Answer from the drawing. Dimensions are ordinates in mm from the lowest x, y and z of the part. A direction names the side the tool comes from. Coordinates: 2 decimals unless noted, no trailing zeros. Loops run counter-clockwise (first coordinate to the right, second up) from the corner with the lowest first, then second, coordinate; pieces in that order, holes last.
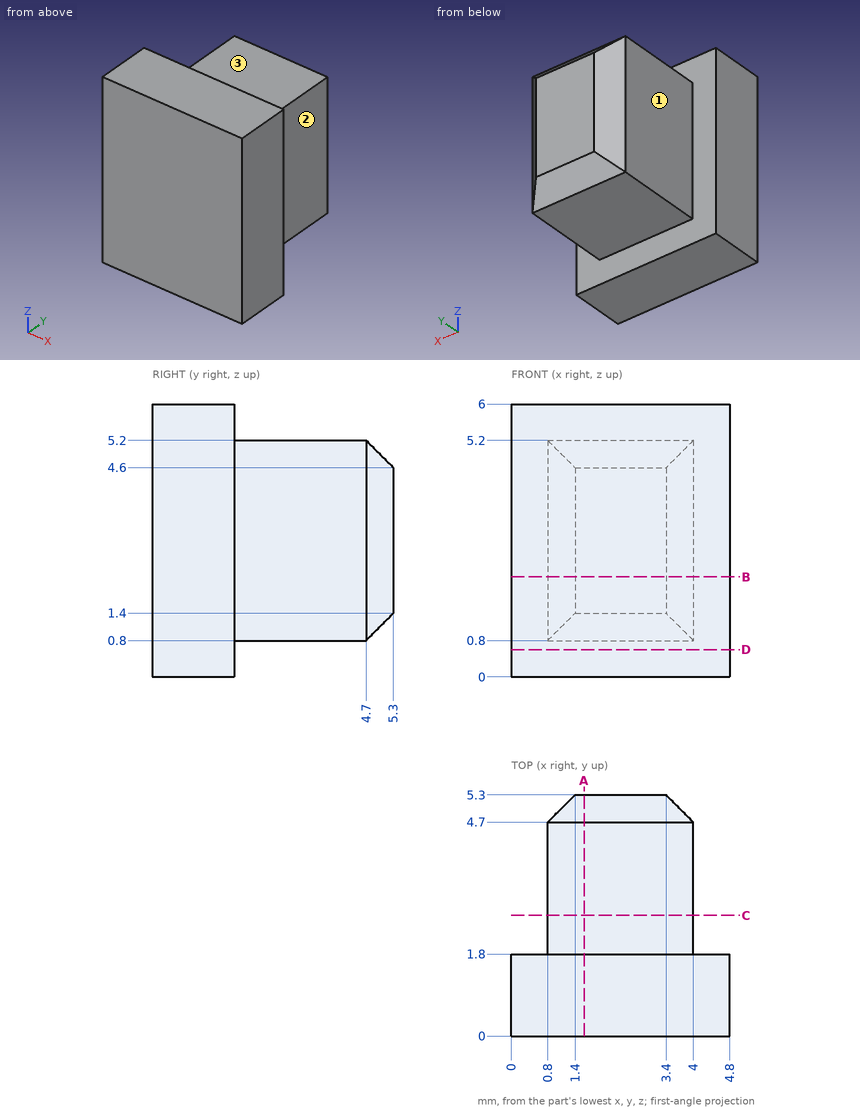
Item 1: Given pin 1 (2 mm diameter, centred on y = 4, z = 5, fed in from +X); pin 2 (0.9 mm diameter, centred on x = 2.5, y = 3.5, fed in from -Z); pin 3 (1.5 mm diameter, centred on x = 3, y = 3, fed in from +Z), each flat-ended and moving along its own axis, determine where each tip first touches the part or whether it passes through.
Numbers:
pin 1: stops at x = 4
pin 2: stops at z = 0.8
pin 3: stops at z = 5.2
Item 2: A cutting plane is placed at D-D on z = 0.6. Determine the outline of the cut face in (x, y), then the cut area to 3 significant figures.
Numbers:
outline: (0, 0) - (4.8, 0) - (4.8, 1.8) - (0, 1.8) - close
area: 8.64 mm2
Item 3: A cutting plane is placed at A-A on x = 1.6. Determine the outline of the cut face in (y, z).
Numbers:
outline: (0, 0) - (1.8, 0) - (1.8, 0.8) - (4.7, 0.8) - (5.3, 1.4) - (5.3, 4.6) - (4.7, 5.2) - (1.8, 5.2) - (1.8, 6) - (0, 6) - close
Item 4: Which of the six approach directions +Z, -Z, +X, -X, +Y, -Y give full straight-line access (tool end or side, diameter ignored) to the marked faces 1, 2 and 3?
Numbers:
face 1: +Z, -Z, -X, +Y
face 2: +Z, -Z, +X, +Y
face 3: +Z, +X, -X, +Y
Item 5: A cutting plane is placed at C-C on y = 2.65. Determine the outline of the cut face in (x, z).
Numbers:
outline: (0.8, 0.8) - (4, 0.8) - (4, 5.2) - (0.8, 5.2) - close
Item 6: A cutting plane is placed at B-B on z = 2.2. Determine the outline of the cut face in (x, y).
Numbers:
outline: (0, 0) - (4.8, 0) - (4.8, 1.8) - (4, 1.8) - (4, 4.7) - (3.4, 5.3) - (1.4, 5.3) - (0.8, 4.7) - (0.8, 1.8) - (0, 1.8) - close
Item 7: Find the intervals of material crossed by line 1 along X through (y, z) = (2.15, 4.5); line 2 along Y through (x, z) = (4.25, 2.85); line 3 along Z through (x, y) = (2.1, 3.35), in increasing order.
Numbers:
line 1: x = 0.8 to 4
line 2: y = 0 to 1.8
line 3: z = 0.8 to 5.2
